```python
from build123d import *

# Parameters (mm, degrees)
TUBE_RECTANGULAR_220_X_140_X_8_0_1_DEPTH = 180
SKETCH_5_R                               = 5.5
CUT_EXTRUDE_1_DEPTH                      = 10
SKETCH_6_R                               = 10
CUT_EXTRUDE_2_DEPTH                      = 10


with BuildPart() as part:
    # Sketch1 → Tube (rectangular) 220 X 140 X 8.0(1) (new body)
    with BuildSketch(Plane(origin=(0, 0, 0), x_dir=(-1, 0, 0), z_dir=(0, 1, 0))):
        with BuildLine():
            Line((-54, -110), (54, -110))
            ThreePointArc((54, -110), (65.313708499, -105.313708499), (70, -94))
            Line((70, -94), (70, 94))
            ThreePointArc((70, 94), (65.313708499, 105.313708499), (54, 110))
            Line((54, 110), (-54, 110))
            ThreePointArc((-54, 110), (-65.313708499, 105.313708499), (-70, 94))
            Line((-70, 94), (-70, -94))
            ThreePointArc((-70, -94), (-65.313708499, -105.313708499), (-54, -110))
        make_face()
        with BuildLine():
            Line((-54, -102), (54, -102))
            ThreePointArc((54, -102), (59.656854249, -99.656854249), (62, -94))
            Line((62, -94), (62, 94))
            ThreePointArc((62, 94), (59.656854249, 99.656854249), (54, 102))
            Line((54, 102), (-54, 102))
            ThreePointArc((-54, 102), (-59.656854249, 99.656854249), (-62, 94))
            Line((-62, 94), (-62, -94))
            ThreePointArc((-62, -94), (-59.656854249, -99.656854249), (-54, -102))
        make_face(mode=Mode.SUBTRACT)
    extrude(amount=TUBE_RECTANGULAR_220_X_140_X_8_0_1_DEPTH)

    # 草图5 → 切除-拉伸1 (cut)
    with BuildSketch(Plane.ZY.offset(70)):
        with Locations((-60, 30)):
            Circle(SKETCH_5_R)
        with Locations((60, 30)):
            Circle(SKETCH_5_R)
        with Locations((-60, 150)):
            Circle(SKETCH_5_R)
        with Locations((60, 150)):
            Circle(SKETCH_5_R)
    extrude(amount=-CUT_EXTRUDE_1_DEPTH, mode=Mode.SUBTRACT)

    # 草图6 → 切除-拉伸2 (cut)
    with BuildSketch(Plane(origin=(70, 0, 0), x_dir=(0, 0, -1), z_dir=(1, 0, 0))):
        with Locations((-60, 150)):
            Circle(SKETCH_6_R)
        with Locations((60, 150)):
            Circle(SKETCH_6_R)
        with Locations((-60, 30)):
            Circle(SKETCH_6_R)
        with Locations((60, 30)):
            Circle(SKETCH_6_R)
    extrude(amount=-CUT_EXTRUDE_2_DEPTH, mode=Mode.SUBTRACT)


solid = part.part
```
Part model, mm, in its own coordinate system. A direction names the side the tool comes from. Coordinates: 2 decimals unless noted, no trailing zeros. Loops run counter-clockwise (first coordinate to the right, second up) from the corner with the lowest first, then second, coordinate; pieces in that order, holes last. Notation, with made-up numbers: (18.25, 55.25) - (73.25, 55.25) arc R24 cw to (73.25, 82.25) - close; hole circle Ø6 at (3, -29). An arc over 180 degrees is marked (long way). Write item = value, one per line. Start each with the question number.
Item 1: Wall check: L1, parallel to Y at x = 67.5, z = 60; L2, parallel to Z at x = -27, y = 109.5; L3, parallel to Y at x = -68, z = 60. Give the ranges that are in metal, low to high. Write a range as from..to.
Item 2: Cut at C-C, the plane y = 112.5. Give the cut face in (x, z).
Item 3: Mould opens along Y. For faces 4 (the flat face through (63, 180, 1)), 5 (the cylindrical face through (66, 24, 68)), 6 (the flat face through (-70, 89, -1)) say: released by +Y, released by -Y, zero draft, split by the parting line, or undercut.
Item 4: Flat gauge pins, fed straight in: pin 1 Ø12.5 at (y, z) = (30, -60) entering from +X; pin 2 Ø23 at (y, z) = (150, -60) entering from +X. Where does each tip first touch, or does it go through?
Item 5: Cut at D-D, the plane x = 43. Give the cut face in (y, z), and give its area (3 significant figures).
Item 6: 3-axis set-ups, long thin cutter, end or side, ignore diameter. For faces 1 (the flat face through (-1, 89, 110)), 2 (the flat face through (-1, 89, 102)), 3 (the cylindrical face through (66.06, 140.24, 62.17)): which of +Z, -Z, +X, -X, +Y, -Y reach the whole face in a straight line?
Item 7: Cut at B-B, the plane z = -45.5. Give the cut face in (x, y), and give its area (3 significant figures).
Item 8: Cut at A-A, the plane y = 150. State how many separate pieces and enclosed holes the cut face has, and give its area (3 significant figures).
The answers:
q1.L1 = 0..20, 40..140, 160..180
q1.L2 = -110..-102, 102..110
q1.L3 = 0..24.5, 35.5..144.5, 155.5..180
q2.outline = (-70, -94) arc R16 ccw to (-54, -110) - (54, -110) arc R16 ccw to (70, -94) - (70, 94) arc R16 ccw to (54, 110) - (-54, 110) arc R16 ccw to (-70, 94) - close; hole (-62, -94) arc R8 ccw to (-54, -102) - (54, -102) arc R8 ccw to (62, -94) - (62, 94) arc R8 ccw to (54, 102) - (-54, 102) arc R8 ccw to (-62, 94) - close
q3.face_4 = released by +Y
q3.face_5 = undercut
q3.face_6 = zero draft
q4.pin_1 = -62
q4.pin_2 = 70
q5.outline = (0, -110) - (180, -110) - (180, -102) - (0, -102) - close; (0, 102) - (180, 102) - (180, 110) - (0, 110) - close
q5.area = 2,880 mm2
q6.face_1 = +Z, +X, -X, +Y, -Y
q6.face_2 = +Y, -Y
q6.face_3 = +X
q7.outline = (-70, 0) - (-62, 0) - (-62, 180) - (-70, 180) - close; (62, 0) - (70, 0) - (70, 180) - (62, 180) - close
q7.area = 2,880 mm2
q8.separate_pieces = 4
q8.enclosed_holes = 0
q8.area = 4,840 mm2
